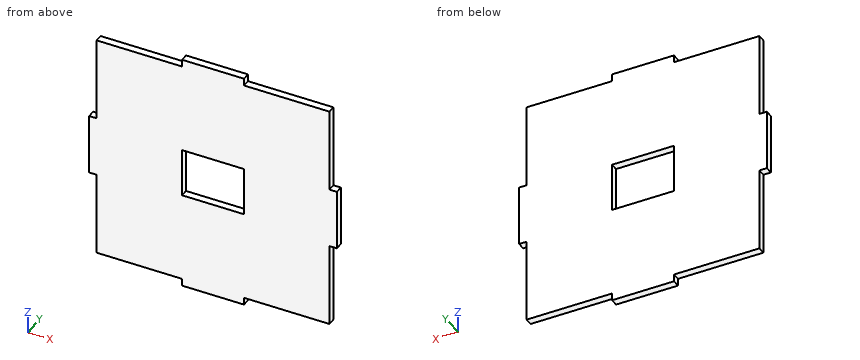
Autodesk Inventor part; units mm, degrees
ref_plane "YZ Plane" through (0, 0, 0) normal (1, 0, 0) x (0, 1, 0)
ref_plane "XZ Plane" through (0, 0, 0) normal (0, 1, 0) x (-1, 0, 0)
ref_plane "XY Plane" through (0, 0, 0) normal (0, 0, 1) x (1, 0, 0)
sketch "Sketch1" plane through (0, 0, 0) normal (0, 1, 0) x (-1, 0, 0)
  line L0 (0, 0) -> (50, 0) construction
  line L1 (0, 0) -> (-50, 0) construction
  line L2 (0, 0) -> (0, 50) construction
  line L3 (0, 0) -> (0, -50) construction
  line L4 (0, -50) -> (12.5, -50)
  line L5 (12.5, -50) -> (12.5, -47)
  line L6 (12.5, -47) -> (47, -47)
  line L7 (47, -47) -> (47, -12.5)
  line L8 (47, -12.5) -> (50, -12.5)
  line L9 (50, -12.5) -> (50, 0)
  line L10 (50, 0) -> (50, 12.5)
  line L11 (50, 12.5) -> (47, 12.5)
  line L12 (47, 12.5) -> (47, 47)
  line L13 (47, 47) -> (12.5, 47)
  line L14 (12.5, 47) -> (12.5, 50)
  line L15 (12.5, 50) -> (-12.5, 50)
  line L16 (-12.5, 50) -> (-12.5, 47)
  line L17 (-12.5, 47) -> (-47, 47)
  line L18 (-47, 47) -> (-47, 12.5)
  line L19 (-47, 12.5) -> (-50, 12.5)
  line L20 (-50, 12.5) -> (-50, -12.5)
  line L21 (-50, -12.5) -> (-47, -12.5)
  line L22 (-47, -12.5) -> (-47, -47)
  line L23 (-47, -47) -> (-12.5, -47)
  line L24 (-12.5, -47) -> (-12.5, -50)
  line L25 (-12.5, -50) -> (0, -50)
  line L26 (0, 0) -> (0, 10) construction
  line L27 (0, 0) -> (0, -10)
  line L28 (0, 0) -> (12.5, 0) construction
  line L29 (12.5, 0) -> (12.5, -10)
  line L30 (12.5, -10) -> (-12.5, -10)
  line L31 (-12.5, -10) -> (-12.5, 10)
  line L32 (-12.5, 10) -> (12.5, 10)
  line L33 (12.5, 10) -> (12.5, 0)
  dimension "d0" = 50
  dimension "d1" = 50
  dimension "d2" = 50
  dimension "d3" = 50
  dimension "d4" = 12.5
  dimension "d5" = 3
  dimension "d6" = 34.5
  dimension "d7" = 34.5
  dimension "d8" = 3
  dimension "d9" = 12.5
  dimension "d10" = 3
  dimension "d11" = 34.5
  dimension "d12" = 34.5
  dimension "d13" = 3
  dimension "d14" = 25
  dimension "d15" = 3
  dimension "d16" = 34.5
  dimension "d17" = 34.5
  dimension "d18" = 3
  dimension "d19" = 25
  dimension "d20" = 3
  dimension "d21" = 34.5
  dimension "d22" = 34.5
  dimension "d23" = 3
  dimension "d24" = 10
  dimension "d25" = 10
  dimension "d26" = 12.5
  dimension "d27" = 10
  dimension "d28" = 25
  dimension "d29" = 20
  dimension "d30" = 25
extrude "Extrusion1" add sketch "Sketch1" along normal blind 3
properties part number "bolongan"
Geometry check sheet. Reference: the model listing, model coordinates, mm. Give positions to 0.01 mm unless a question says otherwise; leave off trailing zeros. Order: outer loops, then holes, each group sorted by start corner. A loop starts at its lowest first (then second) coordinate and runs counter-clockwise, first axis right, second up. Notation, with made-up numbers: M 58,26.5 L 72,26.5 A16 ccw 72,47.5 Z; hole C 43,56.25 d11. An arc over 180 degrees is marked long. Use a Markdown table: item, result.
Item 1: Section check D-D (x = -40.5). Record the cut outline in (y, z).
Answers follow:
| item | result |
|---|---|
| outline | M 0,-47 L 3,-47 L 3,47 L 0,47 Z |
Item 2: Material ranges on line 1 along X through (y, z) = (2.8, -8.5); line 2 along Z through (x, y) = (-8.5, 1.7); line 3 along Z through (x, y) = (-43, 2.85), recorded low to high.
Answers follow:
| item | result |
|---|---|
| line 1 | x = -50 to -12.5, 12.5 to 50 |
| line 2 | z = -50 to -10, 10 to 50 |
| line 3 | z = -47 to 47 |
Item 3: Section check A-A (x = 9.5). Record the cut outline in (y, z), and give its area (3 significant figures).
Answers follow:
| item | result |
|---|---|
| outline | M 0,-50 L 3,-50 L 3,-10 L 0,-10 Z; M 0,10 L 3,10 L 3,50 L 0,50 Z |
| area | 240 mm2 |
Item 4: Section check C-C (y = 0.75). Record the cut outline in (x, z), and give its area (3 significant figures).
Answers follow:
| item | result |
|---|---|
| outline | M -50,-12.5 L -47,-12.5 L -47,-47 L -12.5,-47 L -12.5,-50 L 12.5,-50 L 12.5,-47 L 47,-47 L 47,-12.5 L 50,-12.5 L 50,12.5 L 47,12.5 L 47,47 L 12.5,47 L 12.5,50 L -12.5,50 L -12.5,47 L -47,47 L -47,12.5 L -50,12.5 Z; hole M -12.5,-10 L 12.5,-10 L 12.5,10 L -12.5,10 Z |
| area | 8,640 mm2 |
Item 5: Section check B-B (z = -3). Record the cut outline in (x, y), and give its area (3 significant figures).
Answers follow:
| item | result |
|---|---|
| outline | M -50,0 L -12.5,0 L -12.5,3 L -50,3 Z; M 12.5,0 L 50,0 L 50,3 L 12.5,3 Z |
| area | 225 mm2 |
Item 6: Depth check by flat-ended pin: P1, Ø1, axis at x = 16, y = 2, coming from the +Z side; P2, Ø1.5, axis at x = 15.5, y = 0.5, coming from the -Z side; P3, Ø1.5, axis at y = 1, z = 32, coming from the -X side. Enter the tip coordinate at first touch or a pass-through.
Answers follow:
| item | result |
|---|---|
| P1 | stops at z = 47 |
| P2 | stops at z = -47 |
| P3 | stops at x = -47 |
